The listing builds one solid part. Answer for the finished solid, in the listing's coordinates (mm). Give positions to 0.01 mm unless a question says otherwise; leave off trailing zeros. Write each loop counter-clockwise with the first axis right and the second up, starting at its lowest first coordinate (ties: lowest second). Pieces come first, ordered by that corner, then holes.
Autodesk Inventor part; units mm, degrees
ref_plane "YZ Plane" through (0, 0, 0) normal (1, 0, 0) x (0, 1, 0)
ref_plane "XZ Plane" through (0, 0, 0) normal (0, 1, 0) x (-1, 0, 0)
ref_plane "XY Plane" through (0, 0, 0) normal (0, 0, 1) x (1, 0, 0)
sketch "Sketch1" plane through (0, 0, 0) normal (0, 0, 1) x (1, 0, 0)
  circle A0 centre (0, 0) radius 6.35
  line L0 (-1.6002, 6.1451) -> (-1.6002, 3.8845)
  line L1 (-1.6002, 3.8845) -> (1.6002, 3.8845)
  line L2 (1.6002, 3.8845) -> (1.6002, 6.1451)
  line L3 (0, 0) -> (0, 7.6821)
  dimension "d0" = 12.7
  dimension "d1" = 3.2004
  dimension "d2" = 1.6002
  dimension "d3" = 2.2606
extrude "Extrusion1" add sketch "Sketch1" along normal blind 152.4 contours A0 L0 L1 L2
properties part number ".5in diameter keyed axle"
Item 1: A cutting plane is placed at A-A, the plane x = 0. Give the vertices of the cut face in (y, z), plus the area to 3 significant figures.
Conclusion:
outline: (-6.35, 0) - (3.88, 0) - (3.88, 152.4) - (-6.35, 152.4) - close
area: 1,560 mm2
Item 2: Each of these flat-tipped pins is pushed along its axis until it touches: P1, Ø1.6, axis at x = 0.5, z = 111.5, coming from the +Y side; P2, Ø4, axis at x = -5, z = 125, coming from the +Y side; P3, Ø3, axis at x = -1, y = 4.5, coming from the +Z side; P4, Ø1.8, axis at y = 5, z = 82.5, coming from the +X side. Where does it stop, or does it pass through?
Conclusion:
P1: stops at y = 3.88
P2: stops at y = 5.6
P3: stops at z = 152.4
P4: stops at x = 4.85
Item 3: Consider probe 1 along Y at (x, z) = (0.25, 101); probe 2 along X at (y, z) = (-3.75, 44.5); probe 3 along X at (y, z) = (-3.5, 47). Determine where each line is inside the solid, lowest interval first.
Conclusion:
probe 1: y = -6.35 to 3.88
probe 2: x = -5.12 to 5.12
probe 3: x = -5.3 to 5.3
Item 4: Determine the mould class of faces 1 (the face through (0, 3.884, 75)), 2 (the face through (0, 0, 152.4)), 3 (the face through (0.257, -6.345, 75.133)) for opening direction X: pulls with the +X half, pulls with the -X half, needs draft (parallel to the pull), parting line crosses it, or undercut.
Conclusion:
face 1: undercut
face 2: needs draft
face 3: parting line crosses it
Item 5: A cutting plane is placed at B-B, the plane y = 2. Give the vertices of the cut face in (x, z).
Conclusion:
outline: (-6.03, 0) - (6.03, 0) - (6.03, 152.4) - (-6.03, 152.4) - close
